from build123d import *

# Parameters (mm, degrees)
F1_DEPTH = 17.526
F3_DEPTH = 6.35
F5_D     = 2.7051
F5_DEPTH = 8.73125
F5_TIP   = 0.8126940303
F7_DEPTH = 6.35


with BuildPart() as f1:
    # F0 (on Right) → F1 (new body, symmetric)
    with BuildSketch(Plane.YZ):
        with BuildLine():
            Line((0, 0), (-41.91, 0))
            Line((-41.91, 0), (-41.91, -6.35))
            Line((-41.91, -6.35), (-8.636, -6.35))
            ThreePointArc((-8.636, -6.35), (-7.0195538982, -7.0195538982), (-6.35, -8.636))
            Line((-6.35, -8.636), (-6.35, -38.1))
            Line((-6.35, -38.1), (0, -38.1))
            Line((0, -38.1), (0, 0))
        make_face()
    extrude(amount=F1_DEPTH, both=True)

    # F2 (on face) → F3 (cut, through all)
    with BuildSketch(Plane.XY):
        with BuildLine():
            Line((17.526, -27.178), (17.526, -17.526))
            Line((17.526, -17.526), (-4.826, -17.526))
            ThreePointArc((-4.826, -17.526), (-9.652, -22.352), (-4.826, -27.178))
            Line((-4.826, -27.178), (17.526, -27.178))
        make_face()
    extrude(amount=-F3_DEPTH, mode=Mode.SUBTRACT)

    # F5
    with Locations(Plane.XY):
        with Locations((-11.176, -6.0452), (11.049, -6.0452), (-11.176, -38.4302), (11.049, -38.4302)):
            Hole(F5_D / 2, depth=F5_DEPTH)
            with Locations((0, 0, -(F5_DEPTH + F5_TIP / 2))):  # 118° drill point
                Cone(0, F5_D / 2, F5_TIP, mode=Mode.SUBTRACT)

    # F6 (on face) → F7 (cut, through all)
    with BuildSketch(Plane(origin=(0, 0, 0), x_dir=(-1, 0, 0), z_dir=(0, 1, 0))):
        with BuildLine():
            Line((12.2174, -22.352), (12.2174, -16.002))
            ThreePointArc((12.2174, -16.002), (9.652, -13.4366), (7.0866, -16.002))
            Line((7.0866, -16.002), (7.0866, -22.352))
            ThreePointArc((7.0866, -22.352), (9.652, -24.9174), (12.2174, -22.352))
        make_face()
        with BuildLine():
            Line((-6.8326, -22.352), (-6.8326, -16.002))
            ThreePointArc((-6.8326, -16.002), (-9.398, -13.4366), (-11.9634, -16.002))
            Line((-11.9634, -16.002), (-11.9634, -22.352))
            ThreePointArc((-11.9634, -22.352), (-9.398, -24.9174), (-6.8326, -22.352))
        make_face()
    extrude(amount=-F7_DEPTH, mode=Mode.SUBTRACT)


solid = f1.part
CAD build for the part. Positions are in the model's coordinates, mm. A direction names the side the tool comes from. Coordinates: 2 decimals unless noted, no trailing zeros. Order: outer loops, then holes, each group sorted by start corner. A loop starts at its lowest first (then second) coordinate and runs counter-clockwise, first axis right, second up. Notation, with made-up numbers: (3.5, 42) -> (54.5, 42) arc R25 cw to (54.5, 75) -> close; hole circle Ø6 at (48.5, 21.25). An arc over 180 degrees is marked (long way). Answer in a Markdown table with one row per item.
1) Mould opens along Z. For faces 6 (the face through (-11.23, -5.66, -9.31)), 7 (the face through (-9.708, -3.131, -13.437)), 8 (the face through (-11, -4.704, -4.427)), 9 (the face through (-9.596, -3.131, -24.917)) say: pulls with the +Z half, pulls with the -Z half, needs draft (parallel to the pull), parting line crosses it, or undercut.
Check values:
| item | result |
|---|---|
| face 6 | pulls with the +Z half |
| face 7 | undercut |
| face 8 | needs draft |
| face 9 | undercut |
2) Flat gauge pins, fed straight in: P1, Ø3.5, axis at x = -11.18, y = -6.05, coming from the +Z side; P2, Ø12, axis at x = 4, z = -28, coming from the -Y side; P3, Ø5, axis at x = -14, y = -12.5, coming from the -Z side. Where does each tip first touch, or does it go through?
Check values:
| item | result |
|---|---|
| P1 | z = 0 |
| P2 | y = -6.35 |
| P3 | z = -6.35 |
3) Band-saw the part on A-A (z = -20). List the corners of the cut face in (x, y).
Check values:
| item | result |
|---|---|
| outline | (-17.53, -6.35) -> (-12.22, -6.35) -> (-12.22, 0) -> (-17.53, 0) -> close; (-7.09, -6.35) -> (6.83, -6.35) -> (6.83, 0) -> (-7.09, 0) -> close; (11.96, -6.35) -> (17.53, -6.35) -> (17.53, 0) -> (11.96, 0) -> close |
4) Band-saw the part on B-B (x = 13). List the corners of the cut face in (y, z), and give its area (3 significant figures).
Check values:
| item | result |
|---|---|
| outline | (-41.91, -6.35) -> (-27.18, -6.35) -> (-27.18, 0) -> (-41.91, 0) -> close; (-17.53, -6.35) -> (-8.64, -6.35) arc R2.29 cw to (-6.35, -8.64) -> (-6.35, -38.1) -> (0, -38.1) -> (0, 0) -> (-17.53, 0) -> close |
| area | 408 mm2 |
5) Which spindle directions (+Z, -Z, +X, -X, +Y, -Y) get a long thin tool onto all of the face, cutting with end or side? Do faces 1 (the face through (-12.217, -3, -19)), 2 (the face through (0, -6.35, -23)), 3 (the face through (6, -27.178, -3)), 4 (the face through (-17.526, -15, -3)), 5 (the face through (0, -41.91, -3)). Say none if no direction does.
Check values:
| item | result |
|---|---|
| face 1 | +Y, -Y |
| face 2 | -Z, +X, -X, -Y |
| face 3 | +Z, -Z, +X |
| face 4 | +Z, -Z, -X, +Y, -Y |
| face 5 | +Z, -Z, +X, -X, -Y |
6) Drill centre lines: line 1 (X direction, y = -4, z = -21); line 2 (Y direction, x = -1, z = -25). Where is each one in solid material? Low to high.
Check values:
| item | result |
|---|---|
| line 1 | -17.53 to -12.22, -7.09 to 6.83, 11.96 to 17.53 |
| line 2 | -6.35 to 0 |
7) Band-saw the part on C-C (z = -4.5). List the corners of the cut face in (x, y), and give its area (3 significant figures).
Check values:
| item | result |
|---|---|
| outline | (-17.53, -41.91) -> (17.53, -41.91) -> (17.53, -27.18) -> (-4.83, -27.18) arc R4.83 cw to (-4.83, -17.53) -> (17.53, -17.53) -> (17.53, 0) -> (-17.53, 0) -> close; hole circle Ø2.71 at (-11.18, -38.43); hole circle Ø2.71 at (-11.18, -6.05); hole circle Ø2.71 at (11.05, -38.43); hole circle Ø2.71 at (11.05, -6.05) |
| area | 1,190 mm2 |
8) Band-saw the part on D-D (x = -8). List the corners of the cut face in (y, z).
Check values:
| item | result |
|---|---|
| outline | (-41.91, -6.35) -> (-25.99, -6.35) -> (-25.99, 0) -> (-41.91, 0) -> close; (-18.72, -6.35) -> (-8.64, -6.35) arc R2.29 cw to (-6.35, -8.64) -> (-6.35, -14.04) -> (0, -14.04) -> (0, 0) -> (-18.72, 0) -> close; (-6.35, -38.1) -> (0, -38.1) -> (0, -24.31) -> (-6.35, -24.31) -> close |
